Input: dimensioned drawing with shaded views. Units: mm. Origin: part minimum x, y, z. Round coordinates to 2 decimals unless told otherwise and drop trailing zeros. Order: outer loops, then holes, each group sorted by start corner. A loop starts at its lowest first (then second) coordinate and runs counter-clockwise, first axis right, second up. Notation, with made-up numbers: (75, 50) - (99, 50) arc R9 cw to (99, 56) - close; hole circle Ø9 at (-17, 47). An arc over 180 degrees is marked (long way). Return JSON: item names as keys, results as strings. Group by question number.
1) Ray query, line 1 (Z direction, x = 38.1, y = 5); line 2 (Z direction, x = 42.5, y = 3.25); line 3 (X direction, y = 4.75, z = 7.5). Return the intervals inside material, ascending. Write a range as from..to.
2) Section A-A, the plane x = 38.1. Return loops of the section in (y, z).
3) Section C-C, the plane y = 2. Return loops of the section in (x, z), plus the area to 3 significant figures.
4) Contact query for a flat-ended pin moving along its axis: P1, Ø20.5, axis at x = 38.1, z = 11.89, coming from the -Y side. Output: stop coordinate, or through.
5) Section B-B, the plane z = 13. Return loops of the section in (x, y).
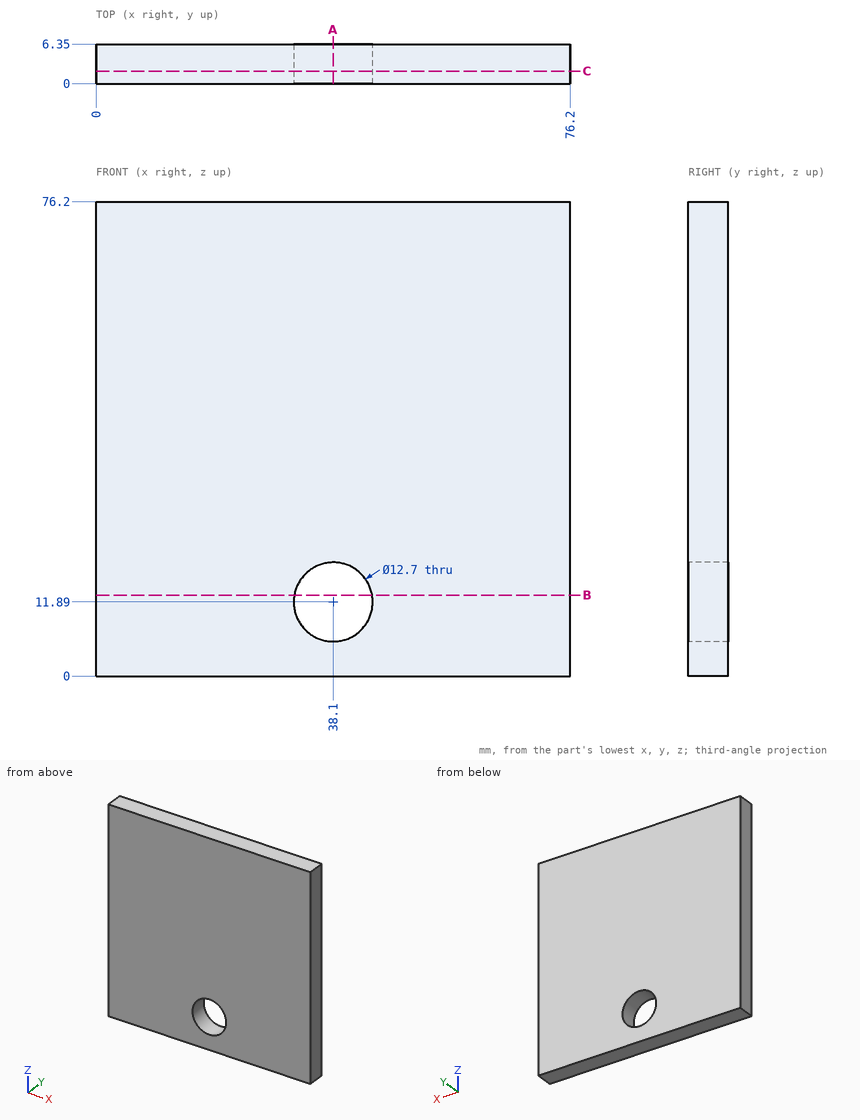
Geometry check:
{
 "1": {"line 1": "0..5.54, 18.24..76.2", "line 2": "0..7.31, 16.47..76.2", "line 3": "0..33.51, 42.69..76.2"},
 "2": {"outline": "(0, 0) - (6.35, 0) - (6.35, 5.54) - (0, 5.54) - close; (0, 18.24) - (6.35, 18.24) - (6.35, 76.2) - (0, 76.2) - close"},
 "3": {"outline": "(0, 0) - (76.2, 0) - (76.2, 76.2) - (0, 76.2) - close; hole circle Ø12.7 at (38.1, 11.89)", "area": "5,680 mm2"},
 "4": {"P1": "y = 0"},
 "5": {"outline": "(0, 0) - (31.85, 0) - (31.85, 6.35) - (0, 6.35) - close; (44.35, 0) - (76.2, 0) - (76.2, 6.35) - (44.35, 6.35) - close"}
}
